```python
from build123d import *

# Parameters (mm, degrees)
SKETCH1_W               = 25.4
SKETCH1_H               = 25.4
BOSS_EXTRUDE1_DEPTH     = 381
SKETCH2_W               = 19.05
SKETCH2_H               = 19.05
CUT_EXTRUDE1_DEPTH      = 1
CUT_EXTRUDE1_DEPTH_BACK = 382


with BuildPart() as part:
    # Sketch1 → Boss-Extrude1 (new body)
    with BuildSketch(Plane(origin=(0, 0, 0), x_dir=(1, 0, 0), z_dir=(0, 1, 0))):
        Rectangle(SKETCH1_W, SKETCH1_H)
    extrude(amount=BOSS_EXTRUDE1_DEPTH)

    # Sketch2 → Cut-Extrude1 (cut, two sides)
    with BuildSketch(Plane(origin=(0, 381, 0), x_dir=(1, 0, 0), z_dir=(0, 1, 0))) as cut_extrude1_sk:
        Rectangle(SKETCH2_W, SKETCH2_H)
    extrude(amount=CUT_EXTRUDE1_DEPTH, mode=Mode.SUBTRACT)
    extrude(cut_extrude1_sk.sketch, amount=-CUT_EXTRUDE1_DEPTH_BACK, mode=Mode.SUBTRACT)


solid = part.part
```
CAD build for the part. Positions are in the model's coordinates, mm. A direction names the side the tool comes from. Round coordinates to 2 decimals unless told otherwise and drop trailing zeros. Order: outer loops, then holes, each group sorted by start corner. A loop starts at its lowest first (then second) coordinate and runs counter-clockwise, first axis right, second up. Notation, with made-up numbers: (-39.5, 88.25) - (-20.5, 88.25) arc R10 ccw to (-20.5, 100.25) - close; hole circle Ø6 at (70, -20.5). An arc over 180 degrees is marked (long way). Use CSV: the item, a comma, the result in double quotes. Start each with the question number.
1) Saw through at A-A (z = -5.5). List the corners of the cut face in (x, y) (3 decimals), and give its area (3 significant figures).
2) Wall check: L1, parallel to X at y = 45.5, z = 0 (3 decimals). Give the ranges that are in metal, low to high. Write a range as [from, to].
3) Tool access for faces 1 (the flat face through (9.525, 193, 0)), 2 (the flat face through (11, 381, 0)): list every direction of +Z, -Z, +X, -X, +Y, -Y with a clear straight run to the whole face (end or side of a thin tool).
4) Two-plate mould, pull along Z, no slides. Class faces 3 (the flat face through (12.7, 188, 0)), 4 (the flat face through (0, 193, -9.525)), 5 (the flat face through (0, 188, -12.7)): pulls with the +Z half, pulls with the -Z half, needs draft (parallel to the pull), parting line crosses it, or undercut.
5) Saw through at C-C (x = 4.5). List the corners of the cut face in (y, z) (3 decimals), and give its area (3 significant figures).
6) Saw through at B-B (y = 264.5). List the corners of the cut face in (x, z) (3 decimals).
Values follow:
1,outline,"(-12.7, 0) - (-9.525, 0) - (-9.525, 381) - (-12.7, 381) - close; (9.525, 0) - (12.7, 0) - (12.7, 381) - (9.525, 381) - close"
1,area,"2,420 mm2"
2,L1,"x = [-12.7, -9.525], [9.525, 12.7]"
3,face 1,"+Y, -Y"
3,face 2,"+Z, -Z, +X, -X, +Y"
4,face 3,"needs draft"
4,face 4,"undercut"
4,face 5,"pulls with the -Z half"
5,outline,"(0, -12.7) - (381, -12.7) - (381, -9.525) - (0, -9.525) - close; (0, 9.525) - (381, 9.525) - (381, 12.7) - (0, 12.7) - close"
5,area,"2,420 mm2"
6,outline,"(-12.7, -12.7) - (12.7, -12.7) - (12.7, 12.7) - (-12.7, 12.7) - close; hole (-9.525, -9.525) - (9.525, -9.525) - (9.525, 9.525) - (-9.525, 9.525) - close"
